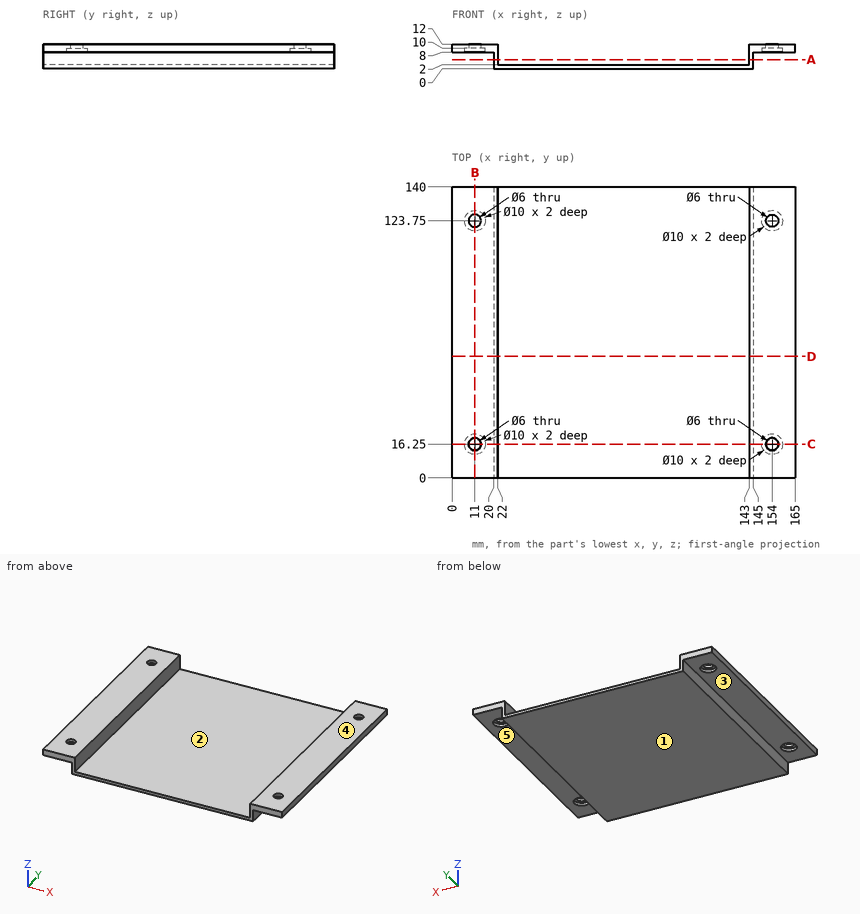
Source: three-view drawing plus pictorial views. Frame: mm from the lowest corner of the part. A direction names the side the tool comes from. Round coordinates to 2 decimals unless told otherwise and drop trailing zeros. Loops run counter-clockwise (first coordinate to the right, second up) from the corner with the lowest first, then second, coordinate; pieces in that order, holes last. Notation, with made-up numbers: (6, 4) - (49, 4) arc R30 cw to (49, 35) - close; hole circle Ø10 at (-23, 34.25). An arc over 180 degrees is marked (long way). Write each question's results on one line, items separated by ' | '. Start each with the question number.
1) Mould query, pull axis X, two halves, no side actions, for the marked faces 1 and 2. Classes: released by +X, released by -X, zero draft, split by the parting line, or undercut.
2) Cut plane B-B on x = 11. Return loops of the section in (y, z), then the cut area to 3 significant figures.
3) Line query: probe 1 along Y at (x, z) = (154, 11.4); probe 2 along X at (y, z) = (123.75, 8.5); probe 3 along X at (y, z) = (123.75, 10.7). Output: solid intervals per line, ascending. Write a range as [from, to].
4) First-contact query: P1, Ø2.5, axis at y = 77.5, z = 2, coming from the -X side; P2, Ø5, axis at x = 155, y = 125, coming from the -Z side; P3, Ø6, axis at x = 160, y = 76.5, coming from the -Z side. Flat tips, straight axial feed; report the tip coordinate or a pass-through.
5) Cut plane C-C on y = 16.25. Return loops of the section in (x, z).
6) Cut plane A-A on z = 4.5. Return loops of the section in (x, y).
7) Access query for the marked faces 3, 4 and 5. Directions: +Z, -Z, +X, -X, +Y, -Y. A direction counts if a zero-diameter tool reaches every point of the face in a straight line with its end or side. Return the directions, or none.
8) Cut plane D-D on y = 58.5. Return loops of the section in (x, z).
Verdict:
1) face 1: zero draft | face 2: undercut
2) outline: (0, 8) - (11.25, 8) - (11.25, 10) - (13.25, 10) - (13.25, 12) - (0, 12) - close; (19.25, 10) - (21.25, 10) - (21.25, 8) - (118.75, 8) - (118.75, 10) - (120.75, 10) - (120.75, 12) - (19.25, 12) - close; (126.75, 10) - (128.75, 10) - (128.75, 8) - (140, 8) - (140, 12) - (126.75, 12) - close | area: 496 mm2
3) probe 1: y = [0, 13.25], [19.25, 120.75], [126.75, 140] | probe 2: x = [0, 6], [16, 22], [143, 149], [159, 165] | probe 3: x = [0, 8], [14, 22], [143, 151], [157, 165]
4) P1: stops at x = 20 | P2: stops at z = 10 | P3: stops at z = 8
5) outline: (0, 8) - (6, 8) - (6, 10) - (8, 10) - (8, 12) - (0, 12) - close; (14, 10) - (16, 10) - (16, 8) - (20, 8) - (20, 0) - (145, 0) - (145, 8) - (149, 8) - (149, 10) - (151, 10) - (151, 12) - (143, 12) - (143, 2) - (22, 2) - (22, 12) - (14, 12) - close; (157, 10) - (159, 10) - (159, 8) - (165, 8) - (165, 12) - (157, 12) - close
6) outline: (20, 0) - (22, 0) - (22, 140) - (20, 140) - close; (143, 0) - (145, 0) - (145, 140) - (143, 140) - close
7) face 3: -Z, -X, +Y, -Y | face 4: +Z, +X, -X, +Y, -Y | face 5: -Z, +X, +Y, -Y
8) outline: (0, 8) - (20, 8) - (20, 0) - (145, 0) - (145, 8) - (165, 8) - (165, 12) - (143, 12) - (143, 2) - (22, 2) - (22, 12) - (0, 12) - close
